Design review of the part built by this model. Coordinates are the model's own, in mm. Face numbers are marked on the shaded views. A direction names the side the tool comes from. Round coordinates to 2 decimals unless told otherwise and drop trailing zeros. Loops run counter-clockwise (first coordinate to the right, second up) from the corner with the lowest first, then second, coordinate; pieces in that order, holes last. Notation, with made-up numbers: (-2.75, 7.25) - (6.25, 7.25) arc R25 ccw to (6.25, 31.25) - close; hole circle Ø4 at (78, 54.25). An arc over 180 degrees is marked (long way). Use one line per item in the form item = value. Start each with the question number.
(1) For pin 1 (2.5 mm diameter, centred on x = 24.5, y = 2, fed in from +Z); pin 2 (10 mm diameter, centred on x = 3.5, y = 1, fed in from +Z); pin 3 (6.5 mm diameter, centred on x = -24, y = 1.5, fed in from +Z), all flat-tipped, find the tip position at first contact; note any pin that passes through.
(2) The part is to be moulded in two halves that separate along Y. For the marked faces 1, 2 and 3, say which applies: released by +Y, released by -Y, zero draft, split by the parting line, or undercut.
(3) We need section B-B, the plane x = 0. Write out the cut boundary in (y, z).
(4) We need section C-C, the plane x = 25. Write out the cut boundary in (y, z), then the cut area to 3 significant figures.
(5) Machinability: for the marked faces 4 and 5, which of the approach directions +Z, -Z, +X, -X, +Y, -Y give a long, thin tool a straight path to every point of the face, cutting with its end or side? Answer none if there is none.
(6) We need section A-A, the plane z = 4.5. Write out the cut boundary in (x, y).
(7) Wall thickness on probe 1 along Y at (x, z) = (-17.2, 8); probe 2 along Y at (x, z) = (0, 8.75); probe 3 along Z at (x, y) = (17.35, 0): over which ranges is each line inside the solid? List them lowest first. Write a range as [from, to].
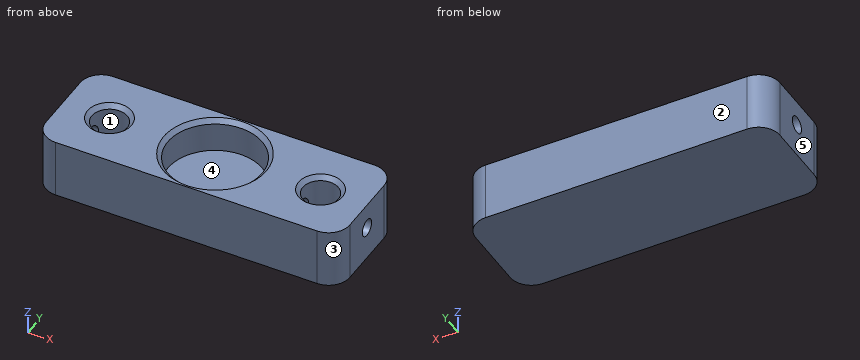
from build123d import *

# Parameters (mm, degrees)
SKETCH1_W               = 72
SKETCH1_H               = 25
BOSS_EXTRUDE1_DEPTH     = 14
SKETCH2_R               = 11.15
CUT_EXTRUDE1_DEPTH      = 8
SKETCH3_R               = 4.2
CUT_EXTRUDE2_DEPTH      = 12
CUT_EXTRUDE3_REACH      = 76.406
CUT_EXTRUDE3_END_RADIUS = 4.2
SKETCH6_R               = 2
ZAOKR_GLENIE1_R         = 5
SFAZOWANIE1_SIZE        = 1


with BuildPart() as part:
    # Sketch1 → Boss-Extrude1 (new body)
    with BuildSketch(Plane.XY):
        Rectangle(SKETCH1_W, SKETCH1_H)
    extrude(amount=BOSS_EXTRUDE1_DEPTH)

    # Sketch2 → Cut-Extrude1 (cut)
    with BuildSketch(Plane.XY.offset(14)):
        Circle(SKETCH2_R)
    extrude(amount=-CUT_EXTRUDE1_DEPTH, mode=Mode.SUBTRACT)

    # Sketch3 → Cut-Extrude2 (cut)
    with BuildSketch(Plane.XY.offset(14)):
        with Locations((-25, 0)):
            Circle(SKETCH3_R)
        with Locations((25, 0)):
            Circle(SKETCH3_R)
    extrude(amount=-CUT_EXTRUDE2_DEPTH, mode=Mode.SUBTRACT)

    # Sketch5 → Ø3.5 (3.5) Diameter Hole1 (revolve, cut)
    with BuildSketch(Plane(origin=(-36, 0, 8), x_dir=(0, 0, 1), z_dir=(0, 1, 0))):
        Polygon((0, 0), (0, 21.051506083), (1.75, 20), (1.75, 0), align=None)
    f_3_5_3_5_diameter_hole1 = revolve(axis=Axis((-42.35, 0, 8), (1, 0, 0)), mode=Mode.SUBTRACT)

    # Cut-Extrude3: up to this cylinder (the profile starts outside it)
    cut_extrude3_end = Plane(origin=(-25, 0, 8), z_dir=(0, 0, 1)) * Cylinder(CUT_EXTRUDE3_END_RADIUS, 162.212, mode=Mode.PRIVATE)
    # Sketch6 → Cut-Extrude3 (cut, up to the surface)
    with BuildSketch(Plane.ZY.offset(36), mode=Mode.PRIVATE) as cut_extrude3_sk1:
        with Locations(Location((8, 0, 0), (0, 0, 270))):
            Circle(SKETCH6_R)
    cut_extrude3_tool1 = extrude(cut_extrude3_sk1.sketch, amount=-CUT_EXTRUDE3_REACH, mode=Mode.PRIVATE) - cut_extrude3_end
    cut_extrude3 = cut_extrude3_tool1.solids().sort_by_distance((-36, 0, 8))[0]
    add(cut_extrude3, mode=Mode.SUBTRACT)

    # Mirror1: Ø3.5 (3.5) Diameter Hole1, Cut-Extrude3 across plane
    add(f_3_5_3_5_diameter_hole1.mirror(Plane(origin=(0, 0, 0), x_dir=(0, 0, 1), z_dir=(1, 0, 0))), mode=Mode.SUBTRACT)
    add(cut_extrude3.mirror(Plane(origin=(0, 0, 0), x_dir=(0, 0, 1), z_dir=(1, 0, 0))), mode=Mode.SUBTRACT)

    # Zaokrąglenie1
    zaokr_glenie1_edges = [part.edges().sort_by_distance(p)[0] for p in [
        (-36, 12.5, 7),
        (36, 12.5, 7),
        (36, -12.5, 7),
        (-36, -12.5, 7),
    ]]
    fillet(zaokr_glenie1_edges, radius=ZAOKR_GLENIE1_R)

    # Sfazowanie1
    sfazowanie1_edges = [part.edges().sort_by_distance(p)[0] for p in [
        (-11.15, 0, 14),
        (-29.2, 0, 14),
        (20.8, 0, 14),
    ]]
    chamfer(sfazowanie1_edges, length=SFAZOWANIE1_SIZE)


solid = part.part
Data:
q1.pin_1 = 2
q1.pin_2 = 6
q1.pin_3 = 13.85
q2.face_1 = undercut
q2.face_2 = released by +Y
q2.face_3 = released by -Y
q3.outline = (-12.5, 0) - (12.5, 0) - (12.5, 14) - (12.15, 14) - (11.15, 13) - (11.15, 6) - (-11.15, 6) - (-11.15, 13) - (-12.15, 14) - (-12.5, 14) - close
q4.outline = (-12.5, 0) - (12.5, 0) - (12.5, 14) - (5.2, 14) - (4.2, 13) - (4.2, 2) - (-4.2, 2) - (-4.2, 13) - (-5.2, 14) - (-12.5, 14) - close
q4.area = 248 mm^2
q5.face_4 = +Z
q5.face_5 = +Z, -Z, -X, +Y, -Y
q6.outline = (-36, -7.5) arc R5 ccw to (-31, -12.5) - (31, -12.5) arc R5 ccw to (36, -7.5) - (36, 7.5) arc R5 ccw to (31, 12.5) - (-31, 12.5) arc R5 ccw to (-36, 7.5) - close; hole circle Ø8.4 at (-25, 0); hole circle Ø8.4 at (25, 0)
q7.probe_1 = [-12.5, -1.75], [1.75, 12.5]
q7.probe_2 = [-12.5, -11.15], [11.15, 12.5]
q7.probe_3 = [0, 6.25], [9.75, 14]
